Geometry check sheet. Reference: the model listing, model coordinates, mm. A direction names the side the tool comes from. Give positions to 0.01 mm unless a question says otherwise; leave off trailing zeros. Order: outer loops, then holes, each group sorted by start corner. A loop starts at its lowest first (then second) coordinate and runs counter-clockwise, first axis right, second up. Notation, with made-up numbers: M 58.5,43.25 L 94.5,43.25 A34 cw 94.5,77.25 Z; hole C 27,76 d8. An arc over 180 degrees is marked long. Answer as CSV lines item,"result".
from build123d import *

# Parameters (mm, degrees)
SKETCH_1_W      = 4
SKETCH_1_H      = 50
EXTRUDE_1_DEPTH = 4


with BuildPart() as part:
    # Эскиз1 → Бобышка-Вытянуть1 (new body)
    with BuildSketch(Plane.XY):
        Polygon((-100, 77.20842051), (-130, 77.20842051), (-130, -22.79157949), (-130, -26.79157949), (-100, -26.79157949), (-100, -22.79157949), (-30, -22.79157949), (-30, -26.79157949), (0, -26.79157949), (4, -26.79157949), (4, 2.20842051), (0, 2.20842051), (0, 52.20842051), (4, 52.20842051), (4, 77.20842051), (0, 77.20842051), (-30, 77.20842051), (-30, 81.20842051), (-100, 81.20842051), align=None)
        with Locations((-28, 27.20842051)):
            Rectangle(SKETCH_1_W, SKETCH_1_H, mode=Mode.SUBTRACT)
    extrude(amount=EXTRUDE_1_DEPTH)


solid = part.part
(1) Section check B-B on y = 16.5. Enter the section's corners in (x, z).
The answers:
outline,"M -130,0 L -30,0 L -30,4 L -130,4 Z; M -26,0 L 0,0 L 0,4 L -26,4 Z"
(2) Section check A-A on z = 0.7. Enter the section's corners in (x, y), then the cut area to 3 significant figures.
The answers:
outline,"M -130,-26.79 L -100,-26.79 L -100,-22.79 L -30,-22.79 L -30,-26.79 L 4,-26.79 L 4,2.21 L 0,2.21 L 0,52.21 L 4,52.21 L 4,77.21 L -30,77.21 L -30,81.21 L -100,81.21 L -100,77.21 L -130,77.21 Z; hole M -30,2.21 L -26,2.21 L -26,52.21 L -30,52.21 Z"
area,"13,500 mm2"
(3) Material ranges on line 1 (X direction, y = 36.5, z = 3.35); line 2 (Y direction, x = -96, z = 0.7); line 3 (Y direction, x = -20, z = 1.5), recorded low to high.
The answers:
line 1,"x = -130 to -30, -26 to 0"
line 2,"y = -22.79 to 81.21"
line 3,"y = -26.79 to 77.21"
(4) Tool access check on faces 4 (the face through (-28, 52.208, 2)), 5 (the face through (2, 2.208, 2)), 6 (the face through (-30, 79, 2)), 7 (the face through (-115, 77.208, 2)). Record the directions out of +Z, -Z, +X, -X, +Y, -Y that give a thin tool (end or side, any length) a straight path to the whole face; none if there is none.
The answers:
face 4,"+Z, -Z"
face 5,"+Z, -Z, +X"
face 6,"+Z, -Z, +X, +Y"
face 7,"+Z, -Z, -X, +Y"
(5) Draft check along Y on faces 1 (the face through (-30, -25, 2)), 2 (the face through (-30, 27, 2)), 3 (the face through (-13, 77.208, 2)). Enter one of: +Y half, -Y half, draft (parallel to the pull), parting line (faces both ways), or undercut.
The answers:
face 1,"draft"
face 2,"undercut"
face 3,"+Y half"
(6) Section check C-C on x = -15.5. Enter the section's corners in (y, z).
The answers:
outline,"M -26.79,0 L 77.21,0 L 77.21,4 L -26.79,4 Z"
(7) Gauge pin test, flat ends, axial feed: P1, Ø2, axis at x = -57.5, z = 2.5, coming from the -Y side; P2, Ø2, axis at x = -121.5, z = 2.5, coming from the +Y side; P3, Ø1.2, axis at y = 35.5, z = 1, coming from the +X side. Record the tip position at first contact, or that the pin passes through.
The answers:
P1,"stops at y = -22.79"
P2,"stops at y = 77.21"
P3,"stops at x = 0"
